```python
from build123d import *

# Parameters (mm, degrees)
SKETCH1_W           = 250
SKETCH1_H           = 125
SKETCH1_W_2         = 230
SKETCH1_H_2         = 115
BOSS_EXTRUDE1_DEPTH = 100
SKETCH3_W           = 250
SKETCH3_H           = 125
SKETCH3_W_2         = 230
SKETCH3_H_2         = 115
SKETCH3_R           = 25
SKETCH3_W_3         = 50
SKETCH3_H_3         = 50
BOSS_EXTRUDE4_DEPTH = 10


with BuildPart() as part:
    # Sketch1 → Boss-Extrude1 (new body)
    with BuildSketch(Plane.XY):
        Rectangle(SKETCH1_W, SKETCH1_H)
        Rectangle(SKETCH1_W_2, SKETCH1_H_2, mode=Mode.SUBTRACT)
    extrude(amount=BOSS_EXTRUDE1_DEPTH)

    # Sketch3 → Boss-Extrude4 (add)
    # profile 1 of 2: a face of its own
    with BuildSketch(Plane.XY.offset(100)):
        Rectangle(SKETCH3_W, SKETCH3_H)
        Rectangle(SKETCH3_W_2, SKETCH3_H_2, mode=Mode.SUBTRACT)
    # profile 2 of 2: a face of its own
    with BuildSketch(Plane.XY.offset(100)):
        Rectangle(SKETCH3_W_2, SKETCH3_H_2)
        with Locations((75, 0)):
            Circle(SKETCH3_R, mode=Mode.SUBTRACT)
        with Locations((-70, 0)):
            Rectangle(SKETCH3_W_3, SKETCH3_H_3, mode=Mode.SUBTRACT)
        Polygon((0, 28.867513459), (25, -14.43375673), (-25, -14.43375673), align=None, mode=Mode.SUBTRACT)
    extrude(amount=BOSS_EXTRUDE4_DEPTH)


solid = part.part
```
Could you check a few things on this model? Use its own coordinates, in mm. A direction names the side the tool comes from. Round coordinates to 2 decimals unless told otherwise and drop trailing zeros. Write each loop counter-clockwise with the first axis right and the second up, starting at its lowest first coordinate (ties: lowest second). Pieces come first, ordered by that corner, then holes. Notation, with made-up numbers: M 34.25,38.5 L 53.25,38.5 A34 ccw 53.25,68.5 Z; hole C 33,73 d5. An arc over 180 degrees is marked long. Answer in a Markdown table with one row per item. Add a question column.
Q1. Will this pin go through, and if not, where does the flat tip stop? pin 1 Ø6 at (x, y) = (89, 14) entering from +Z.
Q2. Imagine slicing it at C-C (y = 0). Please give me the cut outline in (x, z), then the cut area to 3 significant figures.
Q3. If we mould it in two halves opening along Y, with no side actions, what happens to faces 1 (the flat face through (-2, 62.5, 54)), 2 (the flat face through (-125, -1, 54)), 3 (the flat face through (24, 1, 100))? For each: +Y half, -Y half, draft (parallel to the pull), parting line (faces both ways), or undercut.
Q4. Imagine slicing it at B-B (z = 16.5). Please give me the cut outline in (x, y).
Q5. Imagine slicing it at A-A (x = -61.5). Please give me the cut outline in (y, z), then the cut area to 3 significant figures.
Q6. On a 3-axis mill with a long thin cutter (end or side, diameter ignored), from which of +Z, -Z, +X, -X, +Y, -Y can I reach the whole of each face in a straight line? I mean faces 4 (the flat face through (-115, -1, 49)), 5 (the flat face through (-2, -62.5, 54)), 6 (the flat face through (-70, -25, 105)). Say none if no direction works.
Q7. Imagine slicing it at D-D (x = 28). Please give me the cut outline in (y, z).
Q8. If I drill on line 1 (Y direction, x = -2, z = 44); line 2 (Y direction, x = 75, z = 106); line 3 (X direction, y = 55, z = 92), over which ranges is the centre line in solid material (lowest first)? Write a range as from..to.
Values:
| question | item | result |
|---|---|---|
| 1 | pin 1 | through |
| 2 | outline | M -125,0 L -115,0 L -115,100 L -95,100 L -95,110 L -125,110 Z; M -45,100 L -16.67,100 L -16.67,110 L -45,110 Z; M 16.67,100 L 50,100 L 50,110 L 16.67,110 Z; M 100,100 L 115,100 L 115,0 L 125,0 L 125,110 L 100,110 Z |
| 2 | area | 3,170 mm^2 |
| 3 | face 1 | +Y half |
| 3 | face 2 | draft |
| 3 | face 3 | undercut |
| 4 | outline | M -125,-62.5 L 125,-62.5 L 125,62.5 L -125,62.5 Z; hole M -115,-57.5 L 115,-57.5 L 115,57.5 L -115,57.5 Z |
| 5 | outline | M -62.5,0 L -57.5,0 L -57.5,100 L -25,100 L -25,110 L -62.5,110 Z; M 25,100 L 57.5,100 L 57.5,0 L 62.5,0 L 62.5,110 L 25,110 Z |
| 5 | area | 1,750 mm^2 |
| 6 | face 4 | -Z |
| 6 | face 5 | +Z, -Z, +X, -X, -Y |
| 6 | face 6 | +Z, -Z |
| 7 | outline | M -62.5,0 L -57.5,0 L -57.5,100 L 57.5,100 L 57.5,0 L 62.5,0 L 62.5,110 L -62.5,110 Z |
| 8 | line 1 | -62.5..-57.5, 57.5..62.5 |
| 8 | line 2 | -62.5..-25, 25..62.5 |
| 8 | line 3 | -125..-115, 115..125 |
